Geometry: final body of the model. Coordinates: model frame, mm. A direction names the side the tool comes from. Give positions to 0.01 mm unless a question says otherwise; leave off trailing zeros. Write each loop counter-clockwise with the first axis right and the second up, starting at its lowest first coordinate (ties: lowest second). Pieces come first, ordered by that corner, then holes. Notation, with made-up numbers: M 67.25,-34 L 95.25,-34 A37 cw 95.25,4 Z; hole C 23.5,18.25 d10. An arc over 180 degrees is marked long. Use a Markdown table: item, result. Add a question column.
(1) Pin query (flat end, axial travel): pin 1 Ø1.5 at (x, y) = (0.5, -2) entering from +Z; pin 2 Ø8 at (y, z) = (-26, -16) entering from -X; pin 3 Ø0.9 at (x, y) = (1, 28) entering from +Z; pin 4 Ø4.5 at (y, z) = (-22, 0) entering from -X. Return the tip coordinate at first contact, or that it passes through.
(2) Draft query along Z for faces 1 (the cylindrical face through (1.479, 36.847, 0.766)), 2 (the flat face through (1, -29, -9)), 3 (the flat face through (1, 9, -29)). Return one class per face: released by +Z, released by -Z, zero draft, split by the parting line, or undercut.
(3) Reachability of faces 4 (the flat face through (1, -9, -29)), 5 (the flat face through (1, 9, 29)), 6 (the flat face through (1, -9, 29)) from +Z, -Z, +X, -X, +Y, -Y: full face, straight path, thin tool, end or side. Return the list, or none.
(4) Cut plane C-C (x = 1.5). State how many separate pieces and enclosed holes the cut face has, plus the area to 3 significant figures.
(5) Cut plane D-D (z = -13). Output: boundary loops of the cut face in (x, y), plus the area to 3 significant figures.
(6) Cut plane B-B (y = 35). Output: boundary loops of the cut face in (x, z), plus the area to 3 significant figures.
(7) Cut plane A-A (y = -3). Output: boundary loops of the cut face in (x, z), plus the area to 3 significant figures.
(8) Material intervals for L1, parallel to Z at x = 0.9, y = 22; L2, parallel to Z at x = 1.1, y = -26, sorted ascending.
```python
from build123d import *

# Parameters (mm, degrees)
F1_DEPTH = 3


with BuildPart() as f1:
    # F0 (on Right) → F1 (new body)
    with BuildSketch(Plane.YZ):
        with BuildLine():
            Line((-33, 9), (-33, 0))
            Line((-33, 0), (-24, 0))
            ThreePointArc((-24, 0), (-26.6360389693, 6.3639610307), (-33, 9))
        make_face()
        with BuildLine():
            ThreePointArc((-37, 0), (-35, 2), (-33, 0))
            Line((-33, 0), (-33, 9))
            ThreePointArc((-33, 9), (-39.3639610307, 6.3639610307), (-42, 0))
            Line((-42, 0), (-37, 0))
        make_face()
        with BuildLine():
            Line((-24, 0), (-33, 0))
            Line((-33, 0), (-33, -9))
            ThreePointArc((-33, -9), (-26.6360389693, -6.3639610307), (-24, 0))
        make_face()
        with BuildLine():
            Line((-33, -9), (-33, 0))
            ThreePointArc((-33, 0), (-35, -2), (-37, 0))
            Line((-37, 0), (-42, 0))
            ThreePointArc((-42, 0), (-39.3639610307, -6.3639610307), (-33, -9))
        make_face()
        with BuildLine():
            ThreePointArc((-20, 0), (-22, -2), (-24, 0))
            ThreePointArc((-24, 0), (-26.6360389693, -6.3639610307), (-33, -9))
            Line((-33, -9), (-25, -9))
            ThreePointArc((-25, -9), (-13.686291501, -13.686291501), (-9, -25))
            Line((-9, -25), (-9, -33))
            ThreePointArc((-9, -33), (-6.3639610273, -26.6360389659), (9.7e-09, -24))
            ThreePointArc((9.7e-09, -24), (-2, -22.0000000048), (0, -20))
            Line((0, -20), (0, -10))
            ThreePointArc((0, -10), (-7.0710678119, -7.0710678119), (-10, 0))
            Line((-10, 0), (-20, 0))
        make_face()
        with BuildLine():
            ThreePointArc((-33, 9), (-26.6360389693, 6.3639610307), (-24, 0))
            ThreePointArc((-24, 0), (-22, 2), (-20, 0))
            Line((-20, 0), (-10, 0))
            ThreePointArc((-10, 0), (-7.0710678119, 7.0710678119), (0, 10))
            Line((0, 10), (0, 20))
            ThreePointArc((0, 20), (-2, 21.9999999928), (-1.44e-08, 24))
            ThreePointArc((-1.44e-08, 24), (-6.3639610358, 26.6360389744), (-9, 33))
            Line((-9, 33), (-9, 25))
            ThreePointArc((-9, 25), (-13.686291501, 13.686291501), (-25, 9))
            Line((-25, 9), (-33, 9))
        make_face()
        with BuildLine():
            Line((0, 20), (0, 10))
            ThreePointArc((0, 10), (7.0710678119, 7.0710678119), (10, 0))
            Line((10, 0), (20, 0))
            ThreePointArc((20, 0), (22, 2), (24, 0))
            ThreePointArc((24, 0), (26.6360389693, 6.3639610307), (33, 9))
            Line((33, 9), (25, 9))
            ThreePointArc((25, 9), (13.686291501, 13.686291501), (9, 25))
            Line((9, 25), (9, 33))
            ThreePointArc((9, 33), (6.3639610256, 26.6360389642), (-1.44e-08, 24))
            ThreePointArc((-1.44e-08, 24), (1.4142135573, 23.4142135675), (2, 22))
            ThreePointArc((2, 22), (1.4142135624, 20.5857864376), (0, 20))
        make_face()
        with BuildLine():
            ThreePointArc((10, 0), (7.0710678119, -7.0710678119), (0, -10))
            Line((0, -10), (0, -20))
            ThreePointArc((0, -20), (1.4142135624, -20.5857864376), (2, -22))
            ThreePointArc((2, -22), (1.4142135658, -23.414213559), (9.7e-09, -24))
            ThreePointArc((9.7e-09, -24), (6.3639610341, -26.6360389727), (9, -33))
            Line((9, -33), (9, -25))
            ThreePointArc((9, -25), (13.686291501, -13.686291501), (25, -9))
            Line((25, -9), (33, -9))
            ThreePointArc((33, -9), (26.6360389693, -6.3639610307), (24, 0))
            ThreePointArc((24, 0), (22, -2), (20, 0))
            Line((20, 0), (10, 0))
        make_face()
        with BuildLine():
            Line((0, 33), (-9, 33))
            ThreePointArc((-9, 33), (-6.3639610358, 26.6360389744), (-1.44e-08, 24))
            Line((0, 24), (0, 33))
        make_face()
        with BuildLine():
            ThreePointArc((0, 42), (-6.3639610307, 39.3639610307), (-9, 33))
            Line((-9, 33), (0, 33))
            ThreePointArc((0, 33), (-2, 35), (0, 37))
            Line((0, 37), (0, 42))
        make_face()
        with BuildLine():
            Line((0, -33), (-9, -33))
            ThreePointArc((-9, -33), (-6.3639610307, -39.3639610307), (0, -42))
            Line((0, -42), (0, -37))
            ThreePointArc((0, -37), (-2, -35), (0, -33))
        make_face()
        with BuildLine():
            ThreePointArc((9.7e-09, -24), (-6.3639610273, -26.6360389659), (-9, -33))
            Line((-9, -33), (0, -33))
            Line((0, -33), (0, -24))
        make_face()
        with BuildLine():
            ThreePointArc((9, 33), (6.3639610307, 39.3639610307), (0, 42))
            Line((0, 42), (0, 37))
            ThreePointArc((0, 37), (1.4142135624, 36.4142135624), (2, 35))
            ThreePointArc((2, 35), (1.4142135624, 33.5857864376), (0, 33))
            Line((0, 33), (0, 24))
            ThreePointArc((-1.44e-08, 24), (6.3639610256, 26.6360389642), (9, 33))
        make_face()
        with BuildLine():
            Line((0, -37), (0, -42))
            ThreePointArc((0, -42), (6.3639610307, -39.3639610307), (9, -33))
            Line((9, -33), (0, -33))
            ThreePointArc((0, -33), (1.4142135624, -33.5857864376), (2, -35))
            ThreePointArc((2, -35), (1.4142135624, -36.4142135624), (0, -37))
        make_face()
        with BuildLine():
            ThreePointArc((9, -33), (6.3639610341, -26.6360389727), (9.7e-09, -24))
            Line((0, -24), (0, -33))
            Line((0, -33), (9, -33))
        make_face()
        with BuildLine():
            ThreePointArc((33, 9), (26.6360389693, 6.3639610307), (24, 0))
            Line((24, 0), (33, 0))
            ThreePointArc((33, 0), (35, 2), (37, 0))
            Line((37, 0), (42, 0))
            ThreePointArc((42, 0), (39.3639610307, 6.3639610307), (33, 9))
        make_face()
        with BuildLine():
            Line((33, 0), (24, 0))
            ThreePointArc((24, 0), (26.6360389693, -6.3639610307), (33, -9))
            Line((33, -9), (33, 0))
        make_face()
        with BuildLine():
            ThreePointArc((37, 0), (35, -2), (33, 0))
            Line((33, 0), (33, -9))
            ThreePointArc((33, -9), (39.3639610307, -6.3639610307), (42, 0))
            Line((42, 0), (37, 0))
        make_face()
    extrude(amount=F1_DEPTH)


solid = f1.part
```
Answer list:
| question | item | result |
|---|---|---|
| 1 | pin 1 | z = 41.91 |
| 1 | pin 2 | through |
| 1 | pin 3 | z = 9 |
| 1 | pin 4 | x = 0 |
| 2 | face 1 | undercut |
| 2 | face 2 | released by -Z |
| 2 | face 3 | zero draft |
| 3 | face 4 | -Z, +X, -X, -Y |
| 3 | face 5 | +Z, +X, -X, +Y |
| 3 | face 6 | +Z, +X, -X, -Y |
| 4 | separate pieces | 1 |
| 4 | enclosed holes | 9 |
| 4 | area | 2,370 mm² |
| 5 | outline | M 0,-14.42 L 3,-14.42 L 3,14.42 L 0,14.42 Z |
| 5 | area | 86.5 mm² |
| 6 | outline | M 0,-8.77 L 3,-8.77 L 3,-2 L 0,-2 Z; M 0,2 L 3,2 L 3,8.77 L 0,8.77 Z |
| 6 | area | 40.6 mm² |
| 7 | outline | M 0,-41.49 L 3,-41.49 L 3,-9.54 L 0,-9.54 Z; M 0,9.54 L 3,9.54 L 3,41.49 L 0,41.49 Z |
| 7 | area | 192 mm² |
| 8 | L1 | -9.28 to -2, 2 to 9.28 |
| 8 | L2 | -9 to 9 |
